```python
from build123d import *

# Parameters (mm, degrees)
SKETCH008_R           = 43
SKETCH008_R_2         = 4
PAD002_DEPTH          = 12
SKETCH009_R           = 11
POCKET002_DEPTH       = 7
SKETCH010_R           = 3
POCKET003_DEPTH       = 256.426858
POLARPATTERN001_COUNT = 6
SKETCH011_R           = 2.75
POCKET004_DEPTH       = 256.426858
POLARPATTERN002_COUNT = 4


with BuildPart() as part:
    # Sketch008 (on Face1 of ShapeBinder003) → Pad002 (new body)
    with BuildSketch(Plane.XZ.offset(8)):
        Circle(SKETCH008_R)
        Circle(SKETCH008_R_2, mode=Mode.SUBTRACT)
    extrude(amount=PAD002_DEPTH)

    # Sketch009 (on Face3 of Pad002) → Pocket002 (cut)
    with BuildSketch(Plane(origin=(0, -8, 0), x_dir=(1, 0, 0), z_dir=(0, 1, 0))):
        Circle(SKETCH009_R)
    extrude(amount=-POCKET002_DEPTH, mode=Mode.SUBTRACT)

    # Sketch010 (on Face2 of Pocket002) → Pocket003 (cut, through all)
    with BuildSketch(Plane(origin=(0, -8, 0), x_dir=(1, 0, 0), z_dir=(0, 1, 0))):
        with Locations((0, 16)):
            Circle(SKETCH010_R)
    pocket003 = extrude(amount=-POCKET003_DEPTH, mode=Mode.SUBTRACT)

    # PolarPattern001: Pocket003 ×6 about axis
    polarpattern001_axis = Axis((0, -8, 0), (0, 1, 0))
    for i in range(1, POLARPATTERN001_COUNT):
        add(pocket003.rotate(polarpattern001_axis, i * 360 / POLARPATTERN001_COUNT), mode=Mode.SUBTRACT)

    # Sketch011 (on Face2 of PolarPattern001) → Pocket004 (cut, through all)
    with BuildSketch(Plane(origin=(0, -8, 0), x_dir=(1, 0, 0), z_dir=(0, 1, 0))):
        with Locations((0, 38)):
            Circle(SKETCH011_R)
    pocket004 = extrude(amount=-POCKET004_DEPTH, mode=Mode.SUBTRACT)

    # PolarPattern002: Pocket004 ×4 about axis
    polarpattern002_axis = Axis((0, -8, 0), (0, 1, 0))
    for i in range(1, POLARPATTERN002_COUNT):
        add(pocket004.rotate(polarpattern002_axis, i * 360 / POLARPATTERN002_COUNT), mode=Mode.SUBTRACT)


with BuildPart() as part_1:
    # Body003 placement: moved
    add(part.part.moved(Location((0, -30, 0))))


solid = part_1.part
```
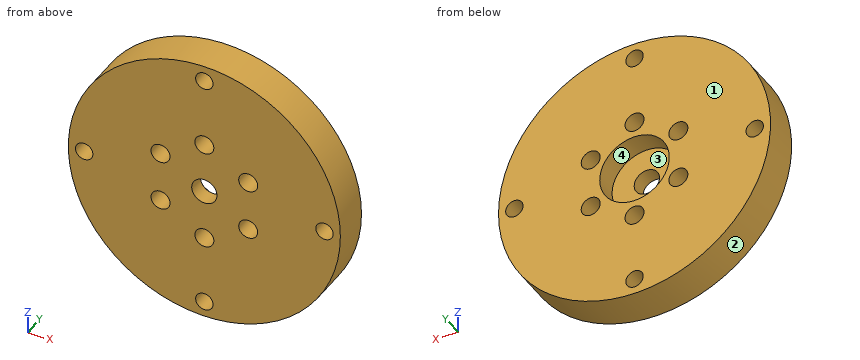
Can you work these out from the model? Positions are in its coordinate system, mm. Face numbers are marked on the shaded views. Coordinates: 2 decimals unless noted, no trailing zeros. Order: outer loops, then holes, each group sorted by start corner. A loop starts at its lowest first (then second) coordinate and runs counter-clockwise, first axis right, second up. Notation, with made-up numbers: (-10.75, 5.25) - (45.25, 5.25) arc R23 cw to (45.25, 25.25) - close; hole circle Ø10 at (36, 82). An arc over 180 degrees is marked (long way). Answer in a Markdown table with one row per item.
1. If I drill on line 1 along Z through (x, y) = (0, -45.5); line 2 along Z through (x, y) = (0, -40.25); line 3 along Z through (x, y) = (-12, -42.5), over which ranges is the centre line in solid material (lowest first)?
Reply:
| item | result |
|---|---|
| line 1 | z = -43 to -40.75, -35.25 to -19, -13 to -4, 4 to 13, 19 to 35.25, 40.75 to 43 |
| line 2 | z = -43 to -40.75, -35.25 to -19, -13 to -11, 11 to 13, 19 to 35.25, 40.75 to 43 |
| line 3 | z = -41.29 to -10.36, -5.64 to 5.64, 10.36 to 41.29 |
2. Suppose I cut it at A-A (x = 0). Please give me the cut outline in (y, z), and give its area (3 significant figures).
Reply:
| item | result |
|---|---|
| outline | (-50, -43) - (-38, -43) - (-38, -40.75) - (-50, -40.75) - close; (-50, -35.25) - (-38, -35.25) - (-38, -19) - (-50, -19) - close; (-50, -13) - (-38, -13) - (-38, -11) - (-45, -11) - (-45, -4) - (-50, -4) - close; (-50, 4) - (-45, 4) - (-45, 11) - (-38, 11) - (-38, 13) - (-50, 13) - close; (-50, 19) - (-38, 19) - (-38, 35.25) - (-50, 35.25) - close; (-50, 40.75) - (-38, 40.75) - (-38, 43) - (-50, 43) - close |
| area | 562 mm^2 |
3. Suppose I cut it at C-C (x = 38). Please give me the cut outline in (y, z), and give its area (3 significant figures).
Reply:
| item | result |
|---|---|
| outline | (-50, -20.12) - (-38, -20.12) - (-38, -2.75) - (-50, -2.75) - close; (-50, 2.75) - (-38, 2.75) - (-38, 20.12) - (-50, 20.12) - close |
| area | 417 mm^2 |
4. If we mould it in two halves opening along Z, with no side actions, what happens to the marked faces 1, 2, 3 and 4? For each: pulls with the +Z half, pulls with the -Z half, needs draft (parallel to the pull), parting line crosses it, or undercut.
Reply:
| item | result |
|---|---|
| face 1 | needs draft |
| face 2 | parting line crosses it |
| face 3 | undercut |
| face 4 | undercut |
5. Suppose I cut it at B-B (z = 1.5). Please give me the cut outline in (x, y).
Reply:
| item | result |
|---|---|
| outline | (-42.97, -50) - (-40.3, -50) - (-40.3, -38) - (-42.97, -38) - close; (-35.7, -50) - (-3.71, -50) - (-3.71, -45) - (-10.9, -45) - (-10.9, -38) - (-35.7, -38) - close; (3.71, -50) - (35.7, -50) - (35.7, -38) - (10.9, -38) - (10.9, -45) - (3.71, -45) - close; (40.3, -50) - (42.97, -50) - (42.97, -38) - (40.3, -38) - close |
6. For pin 1 (5.5 mm diameter, centred on x = 13.86, z = -8, fed in from +Y); pin 2 (11 mm diameter, centred on x = 1.5, z = 3, fed in from +Y); pin 3 (6 mm diameter, centred on x = 18.5, y = -46.5, fed in from +Z), each with a flat end and sliding along its axis, tell me the tip position at first contact or that it passes through.
Reply:
| item | result |
|---|---|
| pin 1 | passes through |
| pin 2 | stops at y = -45 |
| pin 3 | stops at z = 40.11 |
7. Suppose I cut it at D-D (y = -41.5). Give the number of separate pieces and of enclosed holes in the cut face, and give its area (3 significant figures).
Reply:
| item | result |
|---|---|
| separate pieces | 1 |
| enclosed holes | 11 |
| area | 5,160 mm^2 |
